Design review of the part shown in the three views and the two pictorial views. Dimensions are in mm from the part's minimum x, y and z. Coordinates: 2 decimals unless noted, no trailing zeros. Order: outer loops, then holes, each group sorted by start corner. A loop starts at its lowest first (then second) coordinate and runs counter-clockwise, first axis right, second up. Notation, with made-up numbers: (39, -16) -> (45, -16) arc R32 ccw to (45, 16) -> close; hole circle Ø8 at (-22, 60). An arc over 180 degrees is marked (long way). Write item = value, one per line. Start each with the question number.
1) Consider section D-D on x = 35. Give the boundary of the cut face in (y, z) (3 decimals), and give its area (3 significant figures).
2) Consider section B-B on x = 47.5. Give the boundary of the cut face in (y, z) (3 decimals).
3) Consider section A-A on z = 31. Give the boundary of the cut face in (x, y) (3 decimals), and give its area (3 significant figures).
4) Consider section C-C on z = 3. Give the boundary of the cut face in (x, y) (3 decimals).
5) Insertion check: pin 1 Ø2 at (x, z) = (2.5, 31) entering from -Y. The pin has a flat end and moves straight along its axis. Give the tip position at first contact, or say it passes through.
6) Wall thickness on probe 1 along X at (y, z) = (1.4, 31) (3 decimals); probe 2 along X at (y, z) = (1.15, 3); probe 3 along Z at (x, y) = (47.5, 2.05) (3 decimals): over which ranges is each line inside the solid? List them lowest first. Write a range as [from, to].
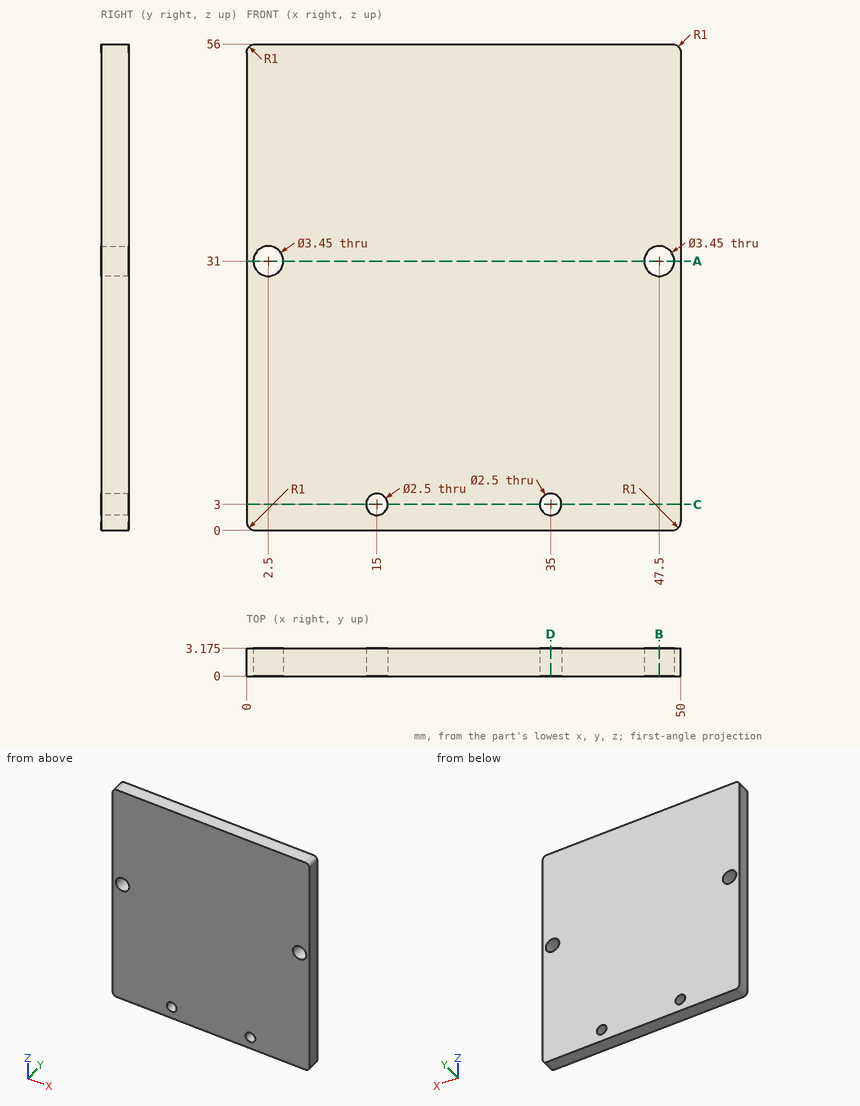
Answer sheet:
q1.outline = (0, 0) -> (3.175, 0) -> (3.175, 1.75) -> (0, 1.75) -> close; (0, 4.25) -> (3.175, 4.25) -> (3.175, 56) -> (0, 56) -> close
q1.area = 170 mm2
q2.outline = (0, 0) -> (3.175, 0) -> (3.175, 29.275) -> (0, 29.275) -> close; (0, 32.725) -> (3.175, 32.725) -> (3.175, 56) -> (0, 56) -> close
q3.outline = (0, 0) -> (0.775, 0) -> (0.775, 3.175) -> (0, 3.175) -> close; (4.225, 0) -> (45.775, 0) -> (45.775, 3.175) -> (4.225, 3.175) -> close; (49.225, 0) -> (50, 0) -> (50, 3.175) -> (49.225, 3.175) -> close
q3.area = 137 mm2
q4.outline = (0, 0) -> (13.75, 0) -> (13.75, 3.175) -> (0, 3.175) -> close; (16.25, 0) -> (33.75, 0) -> (33.75, 3.175) -> (16.25, 3.175) -> close; (36.25, 0) -> (50, 0) -> (50, 3.175) -> (36.25, 3.175) -> close
q5.pin_1 = through
q6.probe_1 = [0, 0.775], [4.225, 45.775], [49.225, 50]
q6.probe_2 = [0, 13.75], [16.25, 33.75], [36.25, 50]
q6.probe_3 = [0, 29.275], [32.725, 56]
